Input: dimensioned drawing with shaded views. Units: mm. Origin: part minimum x, y, z. A direction names the side the tool comes from. Round coordinates to 2 decimals unless told otherwise and drop trailing zeros. Loops run counter-clockwise (first coordinate to the right, second up) from the corner with the lowest first, then second, coordinate; pieces in that order, holes last. Notation, with made-up numbers: (9, -0.75) - (17, -0.75) arc R21 cw to (17, 6.25) - close; hole circle Ø7 at (80, 27.5). An arc over 180 degrees is marked (long way). One line per question, with ' | ' between items.
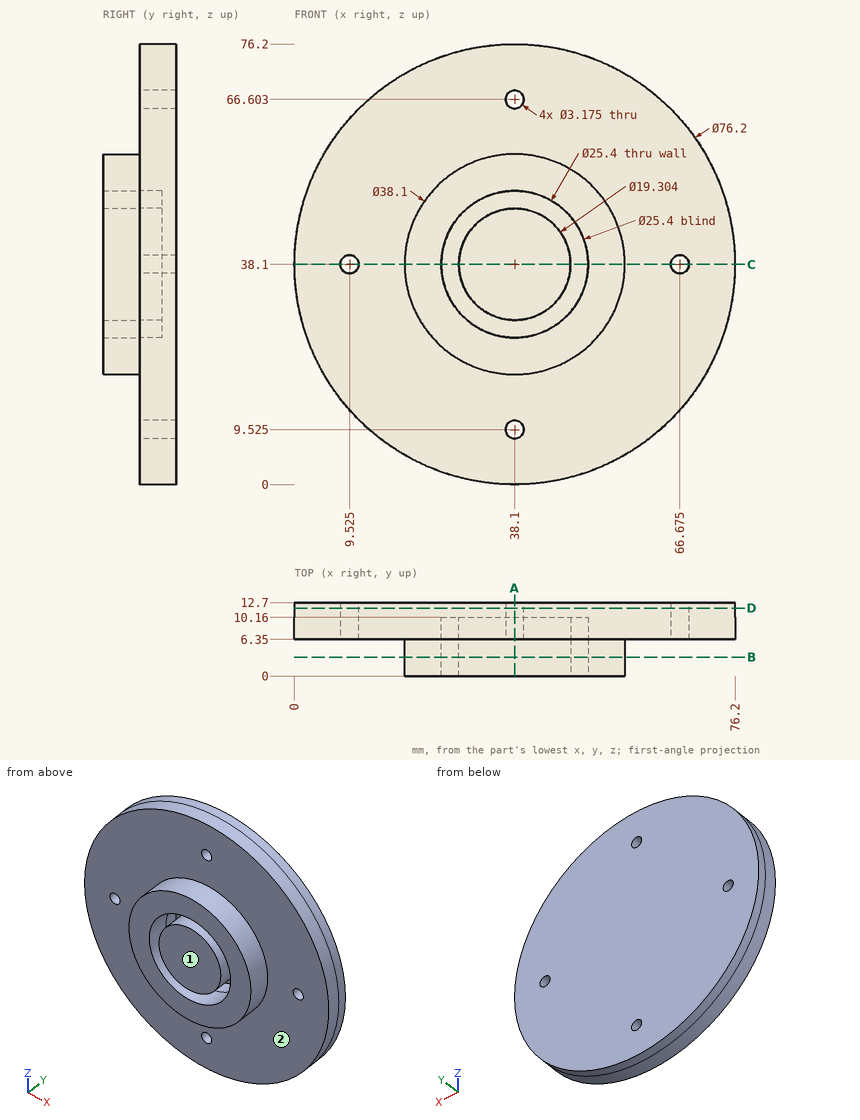
1. Material intervals for probe 1 along Z at (x, y) = (38.1, 8.6); probe 2 along X at (y, z) = (11, 38.1); probe 3 along Z at (x, y) = (38.1, 4.75), sorted ascending.
Worked out:
probe 1: z = 0 to 7.94, 11.11 to 25.4, 28.45 to 47.75, 50.8 to 65.02, 68.19 to 76.2 | probe 2: x = 0 to 7.94, 11.11 to 65.09, 68.26 to 76.2 | probe 3: z = 19.05 to 25.4, 28.45 to 47.75, 50.8 to 57.15
2. Section query B-B, the plane y = 3.25. Return loops of the section in (x, z).
Worked out:
outline: circle Ø38.1 at (38.1, 38.1); circle Ø19.3 at (38.1, 38.1); hole circle Ø25.4 at (38.1, 38.1)
3. Section query A-A, the plane x = 38.1. Return loops of the section in (y, z).
Worked out:
outline: (0, 19.05) - (6.35, 19.05) - (6.35, 11.11) - (12.7, 11.11) - (12.7, 65.02) - (6.35, 65.02) - (6.35, 57.15) - (0, 57.15) - (0, 50.8) - (10.16, 50.8) - (10.16, 47.75) - (0, 47.75) - (0, 28.45) - (10.16, 28.45) - (10.16, 25.4) - (0, 25.4) - close; (6.35, 0) - (12.7, 0) - (12.7, 7.94) - (6.35, 7.94) - close; (6.35, 68.19) - (12.7, 68.19) - (12.7, 76.2) - (6.35, 76.2) - close
4. Access query for the marked faces 1 and 2. Directions: +Z, -Z, +X, -X, +Y, -Y. A direction counts if a zero-diameter tool reaches every point of the face in a straight line with its end or side. Return the directions, or none.
Worked out:
face 1: +Z, -Z, +X, -X, -Y | face 2: -Y
5. Section query C-C, the plane z = 38.1. Return loops of the section in (x, y).
Worked out:
outline: (0, 6.35) - (7.94, 6.35) - (7.94, 12.7) - (0, 12.7) - close; (11.11, 6.35) - (19.05, 6.35) - (19.05, 0) - (25.4, 0) - (25.4, 10.16) - (28.45, 10.16) - (28.45, 0) - (47.75, 0) - (47.75, 10.16) - (50.8, 10.16) - (50.8, 0) - (57.15, 0) - (57.15, 6.35) - (65.09, 6.35) - (65.09, 12.7) - (11.11, 12.7) - close; (68.26, 6.35) - (76.2, 6.35) - (76.2, 12.7) - (68.26, 12.7) - close
6. Section query D-D, the plane y = 11.75. Return loops of the section in (x, z) (1 decimal), plus the area to 3 significant figures.
Worked out:
outline: circle Ø76.2 at (38.1, 38.1); hole circle Ø3.2 at (9.5, 38.1); hole circle Ø3.2 at (38.1, 9.5); hole circle Ø3.2 at (38.1, 66.6); hole circle Ø3.2 at (66.7, 38.1) | area: 4,530 mm2
7. Contact query for flat-ended pins moving along their axis: P1, Ø1.5, axis at x = 12.5, z = 27, coming from the -Y side; P2, Ø4, axis at x = 8.5, y = 10.5, coming from the +Z side (1 decimal); P3, Ø1.5, axis at x = 32.5, y = 7, coming from the +Z side. Output: stop coordinate, or through.
Worked out:
P1: stops at y = 6.35 | P2: stops at z = 64.4 | P3: stops at z = 75.89
